Part model, mm, in its own coordinate system. Round coordinates to 2 decimals unless told otherwise and drop trailing zeros. Write each loop counter-clockwise with the first axis right and the second up, starting at its lowest first coordinate (ties: lowest second). Pieces come first, ordered by that corner, then holes. Notation, with made-up numbers: (-22, 43.25) -> (31, 43.25) arc R29 cw to (31, 64.25) -> close; hole circle Ø5 at (-13, 24). An arc over 180 degrees is marked (long way). Return JSON: item names as keys, results as strings. Group by question number.
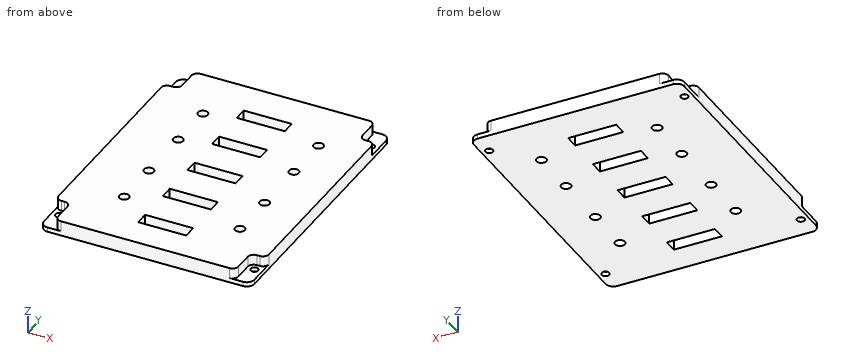
```python
from build123d import *

# Parameters (mm, degrees)
SKETCH1_R           = 3.25
SKETCH1_W           = 32
SKETCH1_H           = 9
BOSS_EXTRUDE1_DEPTH = 10
CUT_EXTRUDE1_DEPTH  = 7
SKETCH3_R           = 2.5
CUT_EXTRUDE2_DEPTH  = 10
FILLET1_R           = 4


with BuildPart() as part:
    # Sketch1 → Boss-Extrude1 (new body)
    with BuildSketch(Plane.XY):
        with BuildLine():
            Line((-67.322274882, 42.630331754), (62.677725118, 42.630331754))
            ThreePointArc((62.677725118, 42.630331754), (66.213259024, 41.165865659), (67.677725118, 37.630331754))
            Line((67.677725118, 37.630331754), (67.677725118, -133.369668246))
            ThreePointArc((67.677725118, -133.369668246), (66.213259024, -136.905202152), (62.677725118, -138.369668246))
            Line((62.677725118, -138.369668246), (-67.322274882, -138.369668246))
            ThreePointArc((-67.322274882, -138.369668246), (-70.857808787, -136.905202152), (-72.322274882, -133.369668246))
            Line((-72.322274882, -133.369668246), (-72.322274882, 37.630331754))
            ThreePointArc((-72.322274882, 37.630331754), (-70.857808787, 41.165865659), (-67.322274882, 42.630331754))
        make_face()
        with Locations((-37.322274882, 4.630331754)):
            Circle(SKETCH1_R, mode=Mode.SUBTRACT)
        with Locations((-37.322274882, -27.369668246)):
            Circle(SKETCH1_R, mode=Mode.SUBTRACT)
        with Locations((-37.322274882, -65.369668246)):
            Circle(SKETCH1_R, mode=Mode.SUBTRACT)
        with Locations((-37.322274882, -97.369668246)):
            Circle(SKETCH1_R, mode=Mode.SUBTRACT)
        with Locations((39.677725118, 4.630331754)):
            Circle(SKETCH1_R, mode=Mode.SUBTRACT)
        with Locations((39.677725118, -27.369668246)):
            Circle(SKETCH1_R, mode=Mode.SUBTRACT)
        with Locations((39.677725118, -65.369668246)):
            Circle(SKETCH1_R, mode=Mode.SUBTRACT)
        with Locations((39.677725118, -97.369668246)):
            Circle(SKETCH1_R, mode=Mode.SUBTRACT)
        with Locations((-1.322274882, 14.130331754)):
            Rectangle(SKETCH1_W, SKETCH1_H, mode=Mode.SUBTRACT)
        with Locations((-1.322274882, -17.869668246)):
            Rectangle(SKETCH1_W, SKETCH1_H, mode=Mode.SUBTRACT)
        with Locations((-1.322274882, -49.869668246)):
            Rectangle(SKETCH1_W, SKETCH1_H, mode=Mode.SUBTRACT)
        with Locations((-1.322274882, -81.869668246)):
            Rectangle(SKETCH1_W, SKETCH1_H, mode=Mode.SUBTRACT)
        with Locations((-1.322274882, -113.869668246)):
            Rectangle(SKETCH1_W, SKETCH1_H, mode=Mode.SUBTRACT)
    extrude(amount=BOSS_EXTRUDE1_DEPTH)

    # Sketch2 → Cut-Extrude1 (cut)
    with BuildSketch(Plane.XY.offset(10)):
        with BuildLine():
            Line((-62.322274882, 42.630331754), (-72.322274882, 42.630331754))
            Line((-72.322274882, 42.630331754), (-72.322274882, 22.630331754))
            Line((-72.322274882, 22.630331754), (-66.322274882, 22.630331754))
            ThreePointArc((-66.322274882, 22.630331754), (-63.493847757, 23.801904629), (-62.322274882, 26.630331754))
            Line((-62.322274882, 26.630331754), (-62.322274882, 42.630331754))
        make_face()
        with BuildLine():
            Line((-72.322274882, -118.369668246), (-66.322274882, -118.369668246))
            ThreePointArc((-66.322274882, -118.369668246), (-63.493847757, -119.541241122), (-62.322274882, -122.369668246))
            Line((-62.322274882, -122.369668246), (-62.322274882, -138.369668246))
            Line((-62.322274882, -138.369668246), (-72.322274882, -138.369668246))
            Line((-72.322274882, -138.369668246), (-72.322274882, -118.369668246))
        make_face()
        with BuildLine():
            Line((57.677725118, -138.369668246), (67.677725118, -138.369668246))
            Line((67.677725118, -138.369668246), (67.677725118, -118.369668246))
            Line((67.677725118, -118.369668246), (61.677725118, -118.369668246))
            ThreePointArc((61.677725118, -118.369668246), (58.849297994, -119.541241122), (57.677725118, -122.369668246))
            Line((57.677725118, -122.369668246), (57.677725118, -138.369668246))
        make_face()
        with BuildLine():
            Line((67.677725118, 22.630331754), (61.677725118, 22.630331754))
            ThreePointArc((61.677725118, 22.630331754), (58.849297994, 23.801904629), (57.677725118, 26.630331754))
            Line((57.677725118, 26.630331754), (57.677725118, 42.630331754))
            Line((57.677725118, 42.630331754), (67.677725118, 42.630331754))
            Line((67.677725118, 42.630331754), (67.677725118, 22.630331754))
        make_face()
    extrude(amount=-CUT_EXTRUDE1_DEPTH, mode=Mode.SUBTRACT)

    # Sketch3 → Cut-Extrude2 (cut)
    with BuildSketch(Plane.XY.offset(3)):
        with Locations((-67.322274882, -123.369668246)):
            Circle(SKETCH3_R)
        with Locations((62.677725118, -123.369668246)):
            Circle(SKETCH3_R)
        with Locations((62.677725118, 27.630331754)):
            Circle(SKETCH3_R)
        with Locations((-67.322274882, 27.630331754)):
            Circle(SKETCH3_R)
    extrude(amount=-CUT_EXTRUDE2_DEPTH, mode=Mode.SUBTRACT)

    # Fillet1
    fillet1_edges = [part.edges().sort_by_distance(p)[0] for p in [
        (57.677725118, 42.630331754, 6.5),
        (67.677725118, 22.630331754, 6.5),
        (67.677725118, -118.369668246, 6.5),
        (57.677725118, -138.369668246, 6.5),
        (-62.322274882, -138.369668246, 6.5),
        (-72.322274882, -118.369668246, 6.5),
        (-72.322274882, 22.630331754, 6.5),
        (-62.322274882, 42.630331754, 6.5),
    ]]
    fillet(fillet1_edges, radius=FILLET1_R)


solid = part.part
```
Item 1: Cut at A-A (x = -5). Write the cut outline in (y, z), then the cut area to 3 significant figures.
Item 2: Cut at C-C (z = 6.5). State how many separate pieces and enclosed holes the cut face has, then the cut area to 3 significant figures.
Item 3: Wall check: L1, parallel to X at y = -96, z = 3.5; L2, parallel to X at y = -20, z = 6.75; L3, parallel to X at y = -99, z = 3.75. Give the ranges that are in metal, low to high.
Item 4: Cut at B-B (y = -52). Write the cut outline in (x, z), then the cut area to 3 significant figures.
Item 5: Flat gauge pins, fed straight in: P1, Ø10.5, axis at x = -37.32, y = -65.37, coming from the -Z side; P2, Ø5.5, axis at y = 31.5, z = 7.5, coming from the +X side; P3, Ø1, axis at x = -67.5, z = 8, coming from the -Y side; P4, Ø4, axis at x = 39.68, y = -27.37, coming from the -Z side. Where does each tip first touch, or does it go through?
Checks:
{
 "1": {"outline": "(-138.37, 0) -> (-118.37, 0) -> (-118.37, 10) -> (-138.37, 10) -> close; (-109.37, 0) -> (-86.37, 0) -> (-86.37, 10) -> (-109.37, 10) -> close; (-77.37, 0) -> (-54.37, 0) -> (-54.37, 10) -> (-77.37, 10) -> close; (-45.37, 0) -> (-22.37, 0) -> (-22.37, 10) -> (-45.37, 10) -> close; (-13.37, 0) -> (9.63, 0) -> (9.63, 10) -> (-13.37, 10) -> close; (18.63, 0) -> (42.63, 0) -> (42.63, 10) -> (18.63, 10) -> close", "area": "1,360 mm2"},
 "2": {"separate pieces": "1", "enclosed holes": "13", "area": "22,800 mm2"},
 "3": {"L1": "x = -72.32 to -40.27, -34.37 to 36.73, 42.63 to 67.68", "L2": "x = -72.32 to -17.32, 14.68 to 67.68", "L3": "x = -72.32 to -40.13, -34.51 to 36.87, 42.49 to 67.68"},
 "4": {"outline": "(-72.32, 0) -> (-17.32, 0) -> (-17.32, 10) -> (-72.32, 10) -> close; (14.68, 0) -> (67.68, 0) -> (67.68, 10) -> (14.68, 10) -> close", "area": "1,080 mm2"},
 "5": {"P1": "stops at z = 0", "P2": "stops at x = 57.68", "P3": "stops at y = -118.37", "P4": "passes through"}
}
